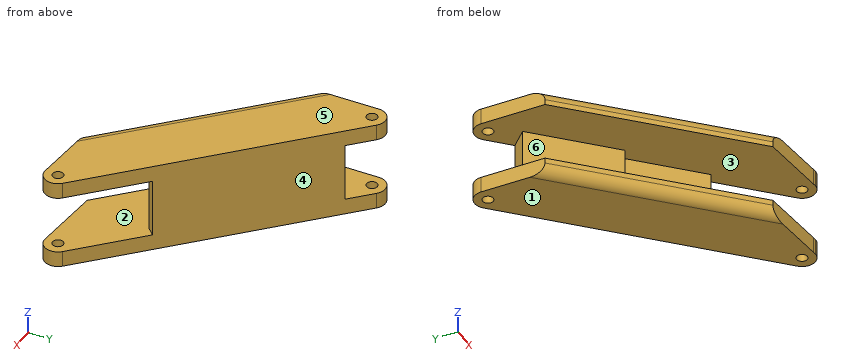
from build123d import *

# Parameters (mm, degrees)
SKETCH1_R           = 1
BOSS_EXTRUDE1_DEPTH = 17
SKETCH2_W           = 17.330300869
SKETCH2_H           = 11
CUT_EXTRUDE1_DEPTH  = 17
SKETCH3_W           = 11
SKETCH3_H           = 11.611712882
CUT_EXTRUDE2_DEPTH  = 64.45501819
SKETCH4_W           = 11
SKETCH4_H           = 15.767820388
BOSS_EXTRUDE2_DEPTH = 2
FILLET1_R           = 2


with BuildPart() as part:
    # Sketch1 → Boss-Extrude1 (new body)
    with BuildSketch(Plane.XY):
        with BuildLine():
            Line((-18.665536599, 40.94089641), (-5.023709167, 27.299068978))
            Line((-5.023709167, 27.299068978), (9.56111442, 12.714245391))
            Line((9.56111442, 12.714245391), (22.179931818, 11.610241922))
            Line((22.179931818, 11.610241922), (22.83879138, 11.552599179))
            ThreePointArc((22.83879138, 11.552599179), (25.056154475, 13.145984205), (24.49310332, 15.817790397))
            Line((24.49310332, 15.817790397), (5.517505351, 34.793388366))
            Line((5.517505351, 34.793388366), (-14.397769646, 54.708663363))
            ThreePointArc((-14.397769646, 54.708663363), (-17.12224518, 55.250595241), (-18.665536599, 52.94089641))
            Line((-18.665536599, 52.94089641), (-18.665536599, 40.94089641))
        make_face()
        with Locations((22.725336367, 14.050023445)):
            Circle(SKETCH1_R, mode=Mode.SUBTRACT)
        with Locations((-16.165536599, 52.94089641)):
            Circle(SKETCH1_R, mode=Mode.SUBTRACT)
    extrude(amount=BOSS_EXTRUDE1_DEPTH)

    # Sketch2 → Cut-Extrude1 (cut)
    with BuildSketch(Plane(origin=(20.155446858, 20.155446858, 0), x_dir=(0.7071067811865516, -0.7071067811865436, 0), z_dir=(0.7071067811865436, 0.7071067811865516, 0))):
        Polygon((-22.401268179, -3), (-25.401268179, -3), (-25.401268179, -14), (31.236683476, -14), (31.236683476, -3), align=None)
        with Locations((-52.031204615, -8.5)):
            Rectangle(SKETCH2_W, SKETCH2_H)
    extrude(amount=-CUT_EXTRUDE1_DEPTH, mode=Mode.SUBTRACT)

    # Sketch3 → Cut-Extrude2 (cut, through all)
    with BuildSketch(Plane(origin=(-30.664430984, 30.664430984, 0), x_dir=(0, 0, 1), z_dir=(-0.7071067811865515, 0.7071067811865437, 0))):
        with Locations((8.5, 18.430482909)):
            Rectangle(SKETCH3_W, SKETCH3_H)
    extrude(amount=-CUT_EXTRUDE2_DEPTH, mode=Mode.SUBTRACT)

    # Sketch4 → Boss-Extrude2 (add)
    with BuildSketch(Plane(origin=(20.155446858, 20.155446858, 0), x_dir=(0, 0, -1), z_dir=(0.7071067811865435, 0.7071067811865516, 0))):
        with Locations((-8.5, 17.517357985)):
            Rectangle(SKETCH4_W, SKETCH4_H)
    extrude(amount=-BOSS_EXTRUDE2_DEPTH)

    # Fillet1
    fillet1_edges = [part.edges().sort_by_distance(p)[0] for p in [
        (-4.55221109, 26.827570901, 17),
        (-4.55221109, 26.827570901, 0),
    ]]
    fillet(fillet1_edges, radius=FILLET1_R)


solid = part.part
Model file for the job. Use its own axes, mm. Face numbers are marked on the shaded views. A direction names the side the tool comes from. Round coordinates to 2 decimals unless told otherwise and drop trailing zeros. Order: outer loops, then holes, each group sorted by start corner. A loop starts at its lowest first (then second) coordinate and runs counter-clockwise, first axis right, second up.
(1) Pin check, flat tips, straight feed: pin 1 (1 mm diameter, centred on y = 44, z = 9.5, fed in from -X); pin 2 (1.8 mm diameter, centred on x = 22.73, y = 14.05, fed in from -Z); pin 3 (4 mm diameter, centred on y = 48, z = 7.5, fed in from +X); pin 4 (3 mm diameter, centred on x = -6.5, z = 11.5, fed in from +Y). Stop position of each tip, or through.
(2) Band-saw the part on A-A (z = 4.5). List the corners of the cut face in (x, y), then the cut area to 3 significant figures.
(3) Drill centre lines: line 1 (Z direction, x = -14, y = 48.5); line 2 (X direction, y = 40.5, z = 6.5); line 3 (X direction, y = 42, z = 13.25). Where is each one in solid material? Low to high.
(4) Pull direction Z, two halves, no side cores. Call the marked faces 1, 2, 3 and 4: released by +Z, released by -Z, zero draft, split by the parting line, or undercut.
(5) 3-axis set-ups, long thin cutter, end or side, ignore diameter. For the marked faces 5 and 6: which of +Z, -Z, +X, -X, +Y, -Y reach the whole face in a straight line?
(6) Band-saw the part on C-C (y = 45.5). List the corners of the cut face in (x, z).
(7) Band-saw the part on B-B (z = 1.25). List the corners of the cut face in (x, y).
Verdict:
1. pin 1: stops at x = -10.22
1. pin 2: passes through
1. pin 3: stops at x = -5.69
1. pin 4: stops at y = 48.31
2. outline: (-13.53, 47.8) - (-0.82, 35.1) - (0.78, 36.7) - (11.93, 25.55) - (13.34, 26.97) - (-10.51, 50.82) - close
2. area: 108 mm2
3. line 1: z = 0 to 3, 14 to 17
3. line 2: x = -6.22 to -0.19
3. line 3: x = -7.72 to -1.69
4. face 1: released by -Z
4. face 2: undercut
4. face 3: undercut
4. face 4: zero draft
5. face 5: +Z, +X, -X, +Y, -Y
5. face 6: -X, -Y
6. outline: (-18.67, 0) - (-5.19, 0) - (-5.19, 17) - (-18.67, 17) - (-18.67, 14) - (-11.22, 14) - (-11.22, 3) - (-18.67, 3) - close
7. outline: (-18.67, 41.15) - (9.79, 12.69) - (22.84, 11.55) arc R2.5 ccw to (24.49, 15.82) - (-14.4, 54.71) arc R2.5 ccw to (-18.67, 52.94) - close; hole circle Ø2 at (-16.17, 52.94); hole circle Ø2 at (22.73, 14.05)
